Part print with two shaded views. Sizes in mm from the minimum x, y, z corner. A direction names the side the tool comes from. Coordinates: 2 decimals unless noted, no trailing zeros. Loops run counter-clockwise (first coordinate to the right, second up) from the corner with the lowest first, then second, coordinate; pieces in that order, holes last.
(1) Two-plate mould, pull along Y, no slides. Class the marked faces 6, 7 and 8: pulls with the +Y half, pulls with the -Y half, needs draft (parallel to the pull), parting line crosses it, or undercut.
(2) Slice it at B-B (x = 69). Give the cut face in (y, z).
(3) Flat gauge pins, fed straight in: P1, Ø1.5, axis at y = 9, z = 19.5, coming from the +X side; P2, Ø10, axis at x = 67.5, y = 22, coming from the +Z side; P3, Ø15.5, axis at y = 16, z = 14.5, coming from the -X side. Where does each tip first touch, or does it go through?
(4) Wall check: L1, parallel to Y at x = 49, z = 5; L2, parallel to X at y = 22.5, z = 6 (1 decimal); L3, parallel to Z at x = 51, y = 42. Give the ranges that are in metal, low to high.
(5) Tool access for the marked faces 1, 2, 3, 4 and 5: list every direction of +Z, -Z, +X, -X, +Y, -Y with a clear straight run to the whole face (end or side of a thin tool).
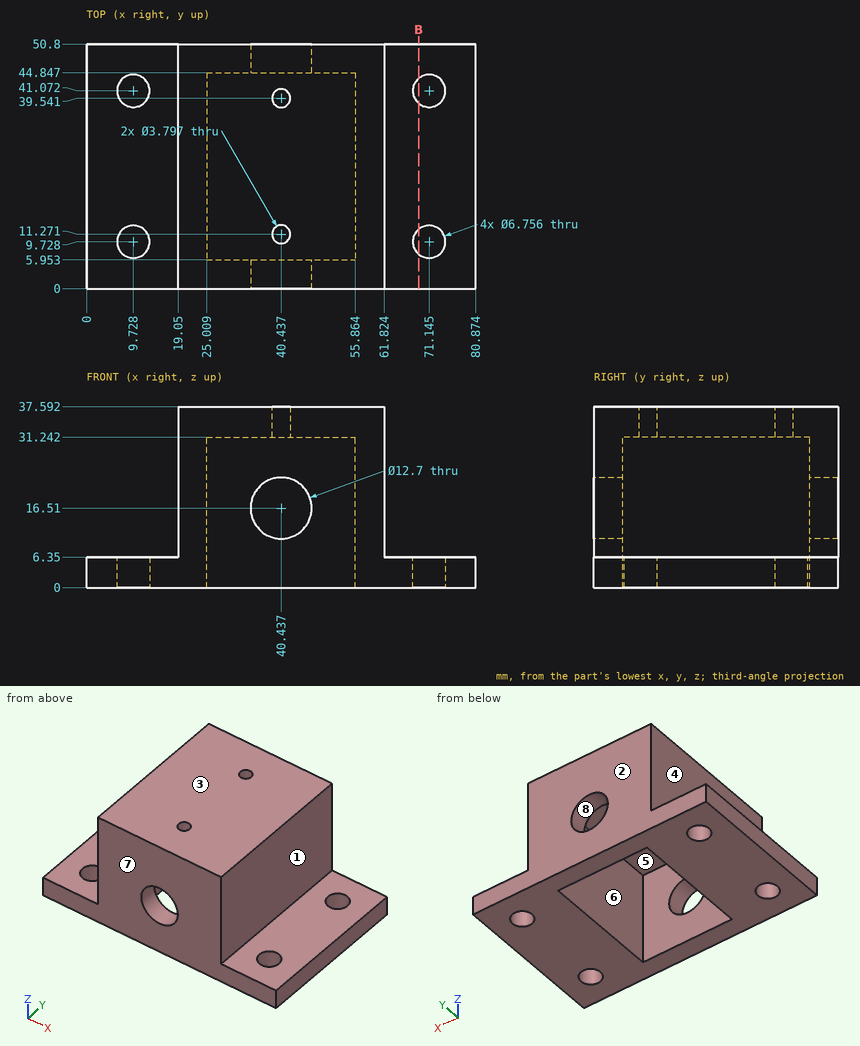
Response values:
1. face 6: undercut
1. face 7: pulls with the -Y half
1. face 8: needs draft
2. outline: (0, 0) - (7.12, 0) - (7.12, 6.35) - (0, 6.35) - close; (12.34, 0) - (38.46, 0) - (38.46, 6.35) - (12.34, 6.35) - close; (43.68, 0) - (50.8, 0) - (50.8, 6.35) - (43.68, 6.35) - close
3. P1: stops at x = 61.82
3. P2: stops at z = 6.35
3. P3: stops at x = 19.05
4. L1: y = 0 to 5.95, 44.85 to 50.8
4. L2: x = 0 to 25, 55.9 to 80.9
4. L3: z = 31.24 to 37.59
5. face 1: +Z, +X, +Y, -Y
5. face 2: +Z, -Z, +X, -X, +Y
5. face 3: +Z, +X, -X, +Y, -Y
5. face 4: +Z, -X, +Y, -Y
5. face 5: -Z
